Print and shaded views of the part. All mm, measured from the part's lowest x, y and z. Coordinates: 2 decimals unless noted, no trailing zeros. Order: outer loops, then holes, each group sorted by start corner. A loop starts at its lowest first (then second) coordinate and runs counter-clockwise, first axis right, second up. Notation, with made-up numbers: M 8,85.25 L 53,85.25 A26 ccw 53,107.25 Z; hole C 68.25,43.25 d5. An arc over 180 degrees is marked long. One line per item, written item: value.
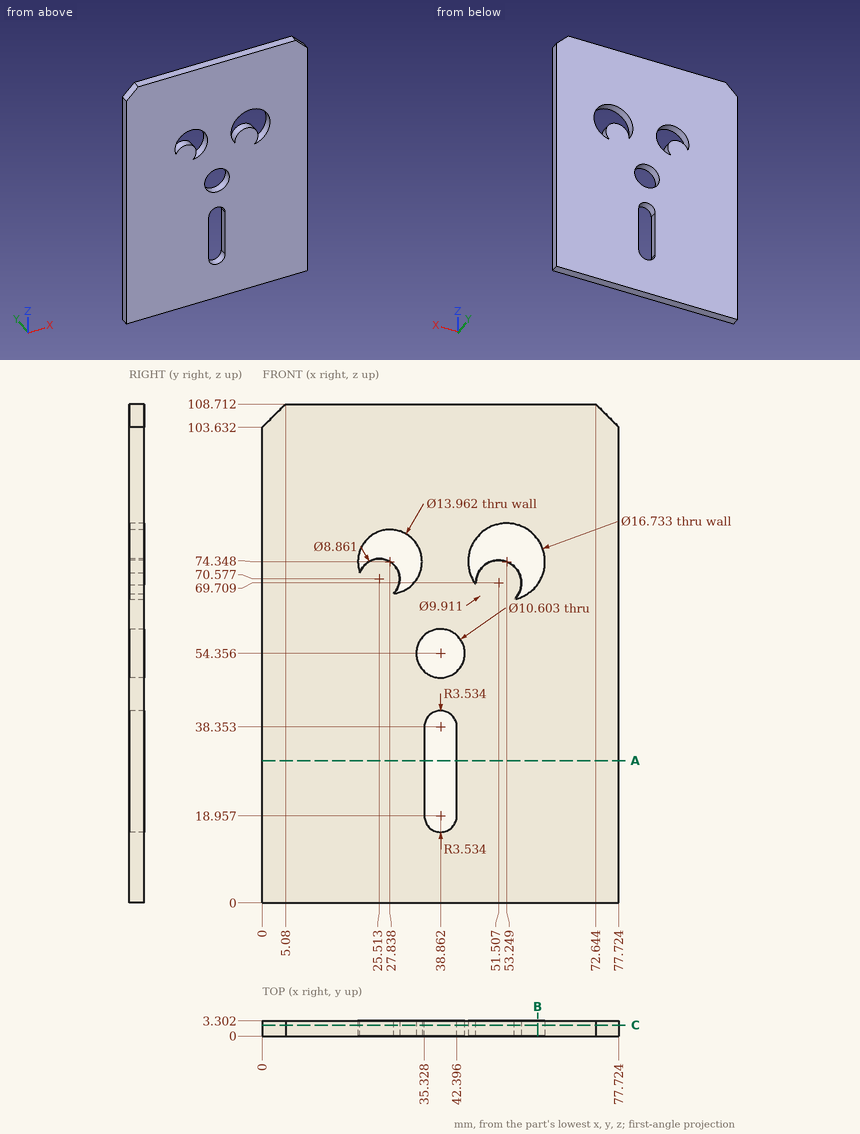
Q1. Slice it at A-A (z = 31). List the corners of the cut face in (x, y).
Recorded:
outline: M 0,0 L 35.33,0 L 35.33,3.3 L 0,3.3 Z; M 42.4,0 L 77.72,0 L 77.72,3.3 L 42.4,3.3 Z
Q2. Drill centre lines: line 1 along X through (y, z) = (2.25, 23.5); line 2 along X through (y, z) = (2.75, 79) (1 decimal); line 3 along X through (y, z) = (0.3, 71) (1 decimal). Where is each one in solid material? Low to high.
Recorded:
line 1: x = 0 to 35.33, 42.4 to 77.72
line 2: x = 0 to 22.6, 33 to 46.3, 60.2 to 77.7
line 3: x = 0 to 29.9, 34 to 45.6, 46.7 to 56.3, 60.9 to 77.7
Q3. Slice it at B-B (x = 60). List the corners of the cut face in (y, z).
Recorded:
outline: M 0,0 L 3.3,0 L 3.3,69.41 L 0,69.41 Z; M 0,79.29 L 3.3,79.29 L 3.3,108.71 L 0,108.71 Z
Q4. Slice it at C-C (y = 2.35). List the corners of the cut face in (x, z) (1 decimal), plus the area to 3 significant figures.
Recorded:
outline: M 0,0 L 77.7,0 L 77.7,103.6 L 72.6,108.7 L 5.1,108.7 L 0,103.6 Z; hole M 21.3,71.9 A4.4 cw long 28.6,67.4 A7 ccw long Z; hole C 38.9,54.4 d10.6; hole M 35.3,19 A3.5 ccw 42.4,19 L 42.4,38.4 A3.5 ccw 35.3,38.4 Z; hole M 46.6,69.3 A5 cw long 55,66.2 A8.4 ccw long Z
area: 7,900 mm^2
